```python
from build123d import *

# Parameters (mm, degrees)
F0_W     = 127
F0_H     = 50.8
F1_DEPTH = 63.5
F2_R     = 50.8
F3_R     = 25.4
F4_DEPTH = 50.801


with BuildPart() as f1:
    # F0 (on Top) → F1 (new body, symmetric)
    with BuildSketch(Plane.XY):
        Rectangle(F0_W, F0_H)
    extrude(amount=F1_DEPTH, both=True)

    # F2
    f2_edges = [f1.edges().sort_by_distance(p)[0] for p in [
        (63.5, 0, 63.5),
    ]]
    fillet(f2_edges, radius=F2_R)

    # F3 (on face) → F4 (cut, through all)
    with BuildSketch(Plane.XZ.offset(25.4)):
        Circle(F3_R)
    extrude(amount=-F4_DEPTH, mode=Mode.SUBTRACT)


solid = f1.part
```
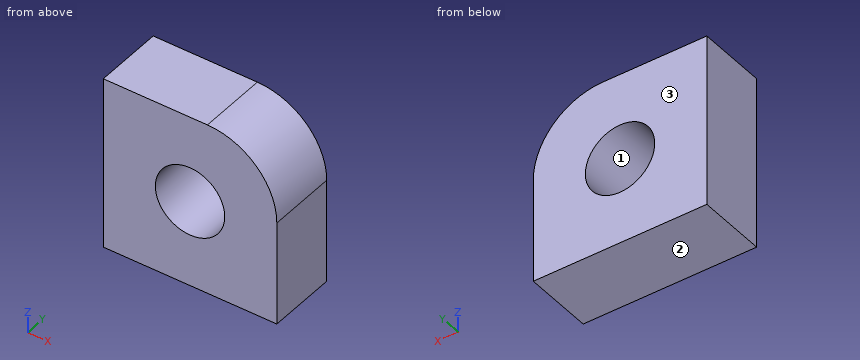
Geometry check sheet. Reference: the model listing, model coordinates, mm. Face numbers are marked on the shaded views. Coordinates: 2 decimals unless noted, no trailing zeros. Order: outer loops, then holes, each group sorted by start corner. A loop starts at its lowest first (then second) coordinate and runs counter-clockwise, first axis right, second up. Notation, with made-up numbers: (72.5, -16) - (118.5, -16) arc R14 ccw to (118.5, 11) - close; hole circle Ø5 at (15.25, 54). An arc over 180 degrees is marked (long way). Answer as a JSON object with one key per item and string values. Group by question number.
Item 1: Scan lines: probe 1 along Z at (x, y) = (0, -14); probe 2 along Z at (x, y) = (18, 12); probe 3 along X at (y, z) = (-11, 3). Record each from-to range of solid material in increasing order.
Item 2: Depth check by flat-ended pin: pin 1 Ø4 at (y, z) = (13, 19.5) entering from +X. Enter the tip coordinate at first touch or a pass-through.
Item 3: Sectioned sample at C-C, the plane x = -7. Record the cut outline in (y, z), and give its area (3 significant figures).
Item 4: Sectioned sample at A-A, the plane z = 0. Record the cut outline in (x, y), and give its area (3 significant figures).
Item 5: Draft check along Z on the marked faces 1, 2 and 3. Enter one of: +Z half, -Z half, draft (parallel to the pull), parting line (faces both ways), or undercut.
Item 6: Sectioned sample at B-B, the plane y = 22. Record the cut outline in (x, z).
Item 7: Sectioned sample at D-D, the plane x = 44.5. Record the cut outline in (y, z), and give its area (3 significant figures).
Resolved:
{
 "1": {"probe 1": "-63.5 to -25.4, 25.4 to 63.5", "probe 2": "-63.5 to -17.92, 17.92 to 63.22", "probe 3": "-63.5 to -25.22, 25.22 to 63.5"},
 "2": {"pin 1": "x = 63.27"},
 "3": {"outline": "(-25.4, -63.5) - (25.4, -63.5) - (25.4, -24.42) - (-25.4, -24.42) - close; (-25.4, 24.42) - (25.4, 24.42) - (25.4, 63.5) - (-25.4, 63.5) - close", "area": "3,970 mm^2"},
 "4": {"outline": "(-63.5, -25.4) - (-25.4, -25.4) - (-25.4, 25.4) - (-63.5, 25.4) - close; (25.4, -25.4) - (63.5, -25.4) - (63.5, 25.4) - (25.4, 25.4) - close", "area": "3,870 mm^2"},
 "5": {"face 1": "undercut", "face 2": "-Z half", "face 3": "draft"},
 "6": {"outline": "(-63.5, -63.5) - (63.5, -63.5) - (63.5, 12.7) arc R50.8 ccw to (12.7, 63.5) - (-63.5, 63.5) - close; hole circle Ø50.8 at (0, 0)"},
 "7": {"outline": "(-25.4, -63.5) - (25.4, -63.5) - (25.4, 52.32) - (-25.4, 52.32) - close", "area": "5,880 mm^2"}
}
